Can you work these out from the model? Positions are in its coordinate system, mm. A direction names the side the tool comes from. Coordinates: 2 decimals unless noted, no trailing zeros. Order: outer loops, then holes, each group sorted by start corner. A loop starts at its lowest first (then second) coordinate and runs counter-clockwise, first axis right, second up. Notation, with made-up numbers: (9, 40.25) -> (43, 40.25) arc R18 cw to (43, 58.25) -> close; hole circle Ø11 at (56.5, 50). An arc over 180 degrees is marked (long way). Answer as CSV lines item,"result".
from build123d import *

# Parameters (mm, degrees)
SKETCH_1_W               = 44
SKETCH_1_H               = 60
EXTRUDE_1_DEPTH          = 19
SKETCH_2_W               = 3
SKETCH_2_H               = 17
CUT_EXTRUDE_1_DEPTH      = 42.773197148
FILLET_1_R               = 3
FILLET_2_R               = 1
SHELL_1_T                = -1.6
EXTRUDE_2_DEPTH          = 17.4
SKETCH_3_3_R             = 0.9
CUT_EXTRUDE_2_DEPTH      = 17.4
MIRROR_2_COPY_1_DEPTH    = 17.4
MIRROR_2_COPY_2_SKETCH_R = 0.9
MIRROR_2_COPY_2_DEPTH    = 17.4
SKETCH_4_W               = 6.8
SKETCH_4_H               = 15
EXTRUDE_3_DEPTH          = 6.2
CUT_EXTRUDE_3_DEPTH      = 42.070183832
CUT_EXTRUDE_3_DEPTH_BACK = 42.070183832
SKETCH_4_4_W             = 2
SKETCH_4_4_H             = 1.7
SKETCH_5_R               = 0.9
EXTRUDE_4_DEPTH          = 6.2
SKETCH_6_W               = 9
SKETCH_6_H               = 3.8
CUT_EXTRUDE_4_DEPTH      = 66.234653368
SKETCH_7_W               = 38
SKETCH_7_H               = 15
CUT_EXTRUDE_5_DEPTH      = 2


with BuildPart() as part:
    # 草图1 → 凸台-拉伸1 (new body)
    with BuildSketch(Plane.XY):
        Rectangle(SKETCH_1_W, SKETCH_1_H)
    extrude(amount=EXTRUDE_1_DEPTH)

    # 草图2 → 切除-拉伸1 (cut, through all)
    with BuildSketch(Plane.XY.offset(19)):
        with Locations((-20.5, 0)):
            Rectangle(SKETCH_2_W, SKETCH_2_H)
        with Locations((20.5, 0)):
            Rectangle(SKETCH_2_W, SKETCH_2_H)
    extrude(amount=-CUT_EXTRUDE_1_DEPTH, mode=Mode.SUBTRACT)

    # 圆角1
    fillet_1_edges = [part.edges().sort_by_distance(p)[0] for p in [
        (22, -30, 9.5),
        (-22, -30, 9.5),
        (-22, 30, 9.5),
        (22, 30, 9.5),
    ]]
    fillet(fillet_1_edges, radius=FILLET_1_R)

    # 圆角2
    fillet_2_edges = [part.edges().sort_by_distance(p)[0] for p in [
        (-19, 8.5, 9.5),
        (-19, -8.5, 9.5),
        (19, -8.5, 9.5),
        (19, 8.5, 9.5),
    ]]
    fillet(fillet_2_edges, radius=FILLET_2_R)

    # 抽壳1
    shell_1_openings = [part.faces().sort_by_distance(p)[0] for p in [
        (0, 0, 19),
    ]]
    offset(amount=SHELL_1_T, openings=shell_1_openings, kind=Kind.INTERSECTION)

    # 草图3 → 凸台-拉伸2 (add)
    with BuildSketch(Plane.XY.offset(1.6)):
        with BuildLine():
            Line((-20.4, 28.4), (-17.9, 28.4))
            ThreePointArc((-17.9, 28.4), (-18.632233047, 26.632233047), (-20.4, 25.9))
            Line((-20.4, 25.9), (-20.4, 28.4))
        make_face()
    extrude_2 = extrude(amount=EXTRUDE_2_DEPTH)

    # 草图3<3> → 切除-拉伸2 (cut)
    with BuildSketch(Plane.XY.offset(1.6)):
        with Locations(Location((-19.9, 27.9, 0), (0, 0, 180))):
            Circle(SKETCH_3_3_R)
    cut_extrude_2 = extrude(amount=CUT_EXTRUDE_2_DEPTH, mode=Mode.SUBTRACT)

    # 镜向1: 凸台-拉伸2, 切除-拉伸2 across plane
    add(extrude_2.mirror(Plane(origin=(0, 0, 0), x_dir=(0, 0, 1), z_dir=(1, 0, 0))))
    add(cut_extrude_2.mirror(Plane(origin=(0, 0, 0), x_dir=(0, 0, 1), z_dir=(1, 0, 0))), mode=Mode.SUBTRACT)

    # 镜向2: 凸台-拉伸2, 切除-拉伸2 across plane
    add(extrude_2.mirror(Plane.ZX))
    add(cut_extrude_2.mirror(Plane.ZX), mode=Mode.SUBTRACT)

    # 镜向2 copy 1 sketch → 镜向2 copy 1 (add)
    with BuildSketch(Plane(origin=(0, 0, 1.6), x_dir=(-1, 0, 0), z_dir=(0, 0, 1))):
        with BuildLine():
            Line((-20.4, 28.4), (-17.9, 28.4))
            ThreePointArc((-17.9, 28.4), (-18.632233047, 26.632233047), (-20.4, 25.9))
            Line((-20.4, 25.9), (-20.4, 28.4))
        make_face()
    extrude(amount=MIRROR_2_COPY_1_DEPTH)

    # 镜向2 copy 2 sketch → 镜向2 copy 2 (cut)
    with BuildSketch(Plane(origin=(0, 0, 1.6), x_dir=(-1, 0, 0), z_dir=(0, 0, 1))):
        with Locations(Location((-19.9, 27.9, 0), (0, 0, 180))):
            Circle(MIRROR_2_COPY_2_SKETCH_R)
    extrude(amount=MIRROR_2_COPY_2_DEPTH, mode=Mode.SUBTRACT)

    # 草图4 → 凸台-拉伸3 (add)
    with BuildSketch(Plane.XY.offset(1.6)):
        with Locations((17, -20.9)):
            Rectangle(SKETCH_4_W, SKETCH_4_H)
    extrude(amount=EXTRUDE_3_DEPTH)

    # 草图4<4> → 切除-拉伸3 (cut, two sides: drawn at the far end of the back side and taken through both)
    with BuildSketch(Plane.XY.offset(1.6).offset(-CUT_EXTRUDE_3_DEPTH_BACK)):
        with Locations((16.2, -26.15)):
            Rectangle(SKETCH_4_4_W, SKETCH_4_4_H)
        with Locations((16.2, -23.61)):
            Rectangle(SKETCH_4_4_W, SKETCH_4_4_H)
        with Locations((16.2, -21.07)):
            Rectangle(SKETCH_4_4_W, SKETCH_4_4_H)
        with Locations((16.2, -18.53)):
            Rectangle(SKETCH_4_4_W, SKETCH_4_4_H)
        with Locations((16.2, -15.99)):
            Rectangle(SKETCH_4_4_W, SKETCH_4_4_H)
    extrude(amount=CUT_EXTRUDE_3_DEPTH + CUT_EXTRUDE_3_DEPTH_BACK, mode=Mode.SUBTRACT)

    # 草图5 → 凸台-拉伸4 (add)
    # profile 1 of 3: a face of its own
    with BuildSketch(Plane.XY.offset(1.6)):
        with BuildLine():
            Line((-17.5, 19.4), (-20.4, 19.4))
            Line((-20.4, 19.4), (-20.4, 15.6))
            Line((-20.4, 15.6), (-17.5, 15.6))
            ThreePointArc((-17.5, 15.6), (-15.6, 17.5), (-17.5, 19.4))
        make_face()
        with Locations(Location((-17.5, 17.5, 0), (0, 0, 180))):
            Circle(SKETCH_5_R, mode=Mode.SUBTRACT)
    # profile 2 of 3: a face of its own
    with BuildSketch(Plane.XY.offset(1.6)):
        with BuildLine():
            Line((20.4, 15.6), (17.5, 15.6))
            ThreePointArc((17.5, 15.6), (15.6, 17.5), (17.5, 19.4))
            Line((17.5, 19.4), (20.4, 19.4))
            Line((20.4, 19.4), (20.4, 15.6))
        make_face()
        with Locations(Location((17.5, 17.5, 0), (0, 0, 180))):
            Circle(SKETCH_5_R, mode=Mode.SUBTRACT)
    # profile 3 of 3: a face of its own
    with BuildSketch(Plane.XY.offset(1.6)):
        with BuildLine():
            Line((-20.4, -15.6), (-17.5, -15.6))
            ThreePointArc((-17.5, -15.6), (-15.6, -17.5), (-17.5, -19.4))
            Line((-17.5, -19.4), (-20.4, -19.4))
            Line((-20.4, -19.4), (-20.4, -15.6))
        make_face()
        with Locations(Location((-17.5, -17.5, 0), (0, 0, 180))):
            Circle(SKETCH_5_R, mode=Mode.SUBTRACT)
    extrude(amount=EXTRUDE_4_DEPTH)

    # 草图6 → 切除-拉伸4 (cut, through all)
    with BuildSketch(Plane(origin=(0, -28.4, 0), x_dir=(1, 0, 0), z_dir=(0, 1, 0))):
        with Locations((0, -11.2)):
            Rectangle(SKETCH_6_W, SKETCH_6_H)
    extrude(amount=-CUT_EXTRUDE_4_DEPTH, mode=Mode.SUBTRACT)

    # 草图7 → 切除-拉伸5 (cut)
    with BuildSketch(Plane(origin=(0, 0, 0), x_dir=(-1, 0, 0), z_dir=(0, 0, -1))):
        Rectangle(SKETCH_7_W, SKETCH_7_H)
    extrude(amount=-CUT_EXTRUDE_5_DEPTH, mode=Mode.SUBTRACT)


solid = part.part
Q1. Imagine slicing it at A-A (x = -14.5). List the corners of the cut face in (y, z) for me, and give its area (3 significant figures).
Solution:
outline,"(-30, 0) -> (-7.5, 0) -> (-7.5, 1.6) -> (-28.4, 1.6) -> (-28.4, 19) -> (-30, 19) -> close; (7.5, 0) -> (30, 0) -> (30, 19) -> (28.4, 19) -> (28.4, 1.6) -> (7.5, 1.6) -> close"
area,"128 mm2"
Q2. Imagine slicing it at B-B (x = -3). List the corners of the cut face in (y, z) for me.
Solution:
outline,"(-30, 0) -> (-7.5, 0) -> (-7.5, 1.6) -> (-28.4, 1.6) -> (-28.4, 9.3) -> (-30, 9.3) -> close; (-30, 13.1) -> (-28.4, 13.1) -> (-28.4, 19) -> (-30, 19) -> close; (7.5, 0) -> (30, 0) -> (30, 19) -> (28.4, 19) -> (28.4, 1.6) -> (7.5, 1.6) -> close"
Q3. Imagine slicing it at C-C (y = 25). List the corners of the cut face in (x, z) for me, and give its area (3 significant figures).
Solution:
outline,"(-22, 0) -> (22, 0) -> (22, 19) -> (20.4, 19) -> (20.4, 1.6) -> (-20.4, 1.6) -> (-20.4, 19) -> (-22, 19) -> close"
area,"126 mm2"
Q4. For P1, Ø10, axis at x = -7.5, y = 3.5, coming from the +Z side; P2, Ø1.6, axis at x = 21, z = 9, coming from the -Y side; P3, Ø1.9, axis at x = -18, y = 17.5, coming from the +Z side, each with a flat end and sliding along its axis, tell me the tip position at first contact or that it passes through.
Solution:
P1,"z = 1.6"
P2,"y = -29.75"
P3,"z = 7.8"
Q5. If I drill on line 1 (X direction, y = -17.5, z = 3.25); line 2 (X direction, y = 17.5, z = 4.5); line 3 (X direction, y = 10.5, z = 2), over which ranges is the centre line in solid material (lowest first)?
Solution:
line 1,"-22 to -18.4, -16.6 to -15.6, 13.6 to 22"
line 2,"-22 to -18.4, -16.6 to -15.6, 15.6 to 16.6, 18.4 to 22"
line 3,"-22 to -20.4, 20.4 to 22"
Q6. Which directions (+Z, -Z, +X, -X, +Y, -Y) give clear straight access to the entire face, cutting with the end or side of a thin tool? Please do faces 3 (the flat face through (-20.4, -18, 10)), 4 (the flat face through (16, -19.38, 4)), 5 (the flat face through (0, 19, 0)).
Solution:
face 3,"+Z"
face 4,"+Z, -Z"
face 5,"-Z, +X, -X, +Y, -Y"
Q7. We'd pull the mould along X, two halves only. Please class faces 1 (the flat face through (-21, -8.5, 10)), 2 (the flat face through (13.6, -21, 5)): pulls with the +X half, pulls with the -X half, needs draft (parallel to the pull), parting line crosses it, or undercut.
Solution:
face 1,"needs draft"
face 2,"undercut"
Q8. Imagine slicing it at D-D (z = 16.5). Give the number of separate pieces and of enclosed holes in the cut face, and give its area (3 significant figures).
Solution:
separate pieces,"1"
enclosed holes,"5"
area,"339 mm2"
